For this review, use the dimensioned drawing (mm, ordinates from the lowest corner) and the shaded views. A direction names the side the tool comes from. Give positions to 0.01 mm unless a question says otherwise; leave off trailing zeros. Write each loop counter-clockwise with the first axis right and the second up, starting at its lowest first coordinate (ties: lowest second). Pieces come first, ordered by that corner, then holes. Notation, with made-up numbers: M 71,-38 L 87,-38 A7 ccw 87,-33 Z; hole C 20,54 d3. An arc over 180 degrees is marked long. Answer in a Markdown table with one row per item.
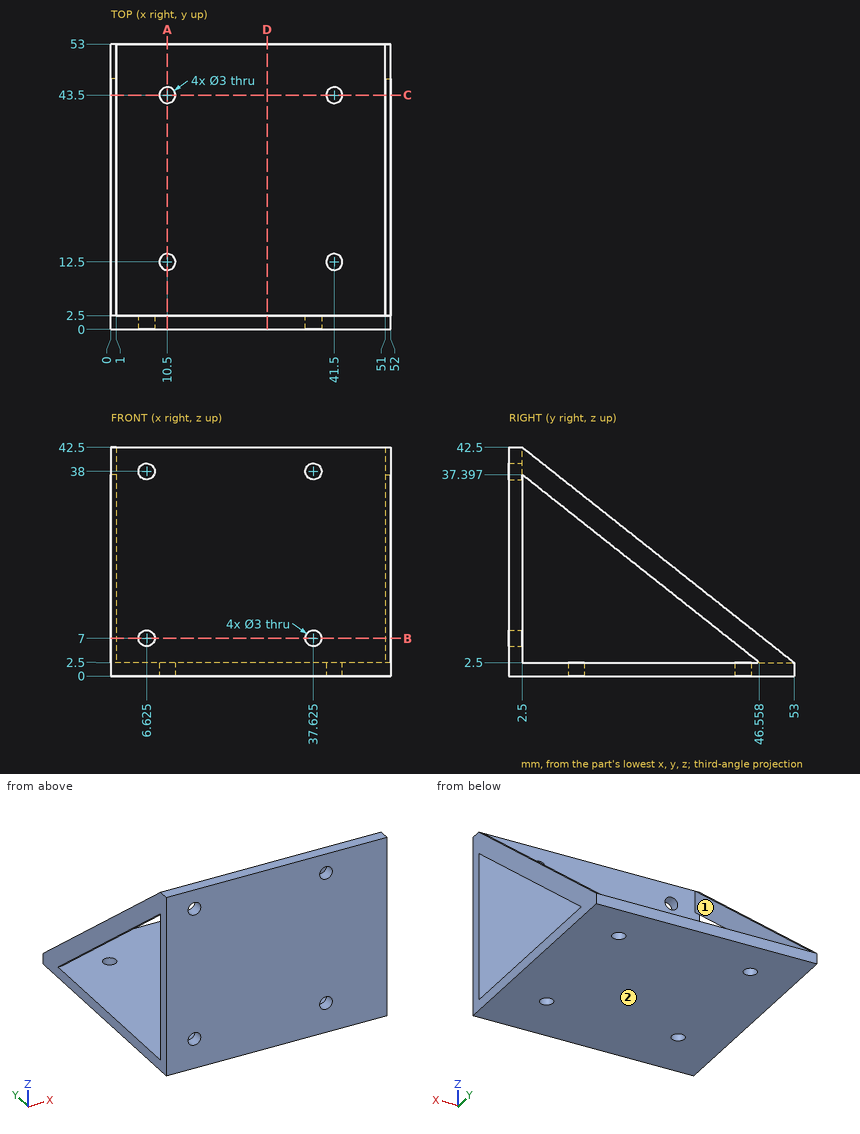
1) Add section B-B (z = 7). Write out the cut boundary in (x, y) (1 decimal).
Geometry says:
| item | result |
|---|---|
| outline | M 0,0 L 5.1,0 L 5.1,2.5 L 0,2.5 Z; M 0,40.9 L 1,40.9 L 1,47.3 L 0,47.3 Z; M 8.1,0 L 36.1,0 L 36.1,2.5 L 8.1,2.5 Z; M 39.1,0 L 52,0 L 52,2.5 L 39.1,2.5 Z; M 51,40.9 L 52,40.9 L 52,47.3 L 51,47.3 Z |
2) Insertion check: P1, Ø5, axis at x = 41.5, y = 12.5, coming from the +Z side; P2, Ø20, axis at x = 33, z = 24, coming from the +Y side; P3, Ø12, axis at x = 45.5, y = 36.5, coming from the +Z side. Each pin has a flat end and moves straight along its axis. Give the tip position at first contact, or say it passes through.
Geometry says:
| item | result |
|---|---|
| P1 | z = 2.5 |
| P2 | y = 2.5 |
| P3 | z = 17.47 |
3) Add section A-A (x = 10.5). Write out the cut boundary in (y, z).
Geometry says:
| item | result |
|---|---|
| outline | M 0,0 L 11,0 L 11,2.5 L 2.5,2.5 L 2.5,42.5 L 0,42.5 Z; M 14,0 L 42,0 L 42,2.5 L 14,2.5 Z; M 45,0 L 53,0 L 53,2.5 L 45,2.5 Z |
4) Add section C-C (y = 43.5). Write out the cut boundary in (x, z) (1 decimal).
Geometry says:
| item | result |
|---|---|
| outline | M 0,0 L 9,0 L 9,2.5 L 0,2.5 Z; M 0,4.9 L 1,4.9 L 1,10 L 0,10 Z; M 12,0 L 40,0 L 40,2.5 L 12,2.5 Z; M 43,0 L 52,0 L 52,2.5 L 43,2.5 Z; M 51,4.9 L 52,4.9 L 52,10 L 51,10 Z |
5) Add section D-D (x = 29). Write out the cut boundary in (y, z).
Geometry says:
| item | result |
|---|---|
| outline | M 0,0 L 53,0 L 53,2.5 L 2.5,2.5 L 2.5,42.5 L 0,42.5 Z |
6) To check wall thickness, follow probe 1 along X at (y, z) = (1.15, 7) (1 decimal); probe 2 along Y at (x, z) = (41.5, 0.85); probe 3 along Y at (x, z) = (10, 1) (1 decimal). State the ranges of each line that lie inside material, in increasing order. Write a range as [from, to].
Geometry says:
| item | result |
|---|---|
| probe 1 | [0, 5.1], [8.1, 36.1], [39.1, 52] |
| probe 2 | [0, 11], [14, 42], [45, 53] |
| probe 3 | [0, 11.1], [13.9, 42.1], [44.9, 53] |
7) For the marked faces 1 and 2, list the 3-axis set-ups (+Z, -Z, +X, -X, +Y, -Y) from which the entire face can be reached by the end or side of a thin tool; tool diameter is ignored.
Geometry says:
| item | result |
|---|---|
| face 1 | +Z, +Y |
| face 2 | -Z, +X, -X, +Y, -Y |
